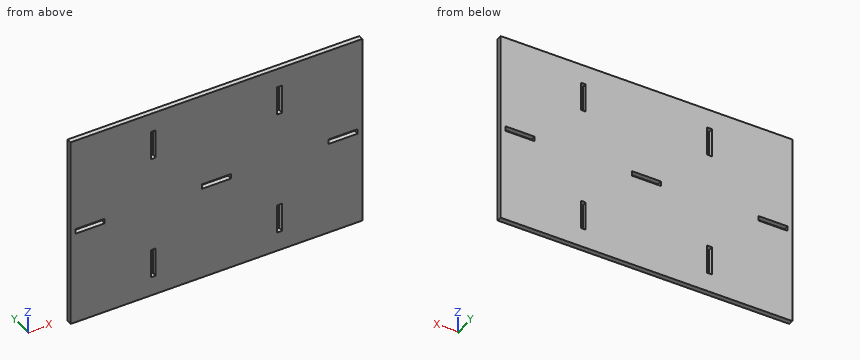
```python
from build123d import *

# Parameters (mm, degrees)
SKETCH1_W           = 300
SKETCH1_H           = 200
BOSS_EXTRUDE1_DEPTH = 5
SKETCH2_W           = 30
SKETCH2_H           = 5
SKETCH2_W_2         = 5
SKETCH2_H_2         = 30
CUT_EXTRUDE1_DEPTH  = 5


with BuildPart() as part:
    # Sketch1 → Boss-Extrude1 (new body)
    with BuildSketch(Plane(origin=(0, 0, 0), x_dir=(1, 0, 0), z_dir=(0, 1, 0))):
        Rectangle(SKETCH1_W, SKETCH1_H)
    extrude(amount=BOSS_EXTRUDE1_DEPTH)

    # Sketch2 → Cut-Extrude1 (cut)
    with BuildSketch(Plane(origin=(0, 5, 0), x_dir=(1, 0, 0), z_dir=(0, 1, 0))):
        with Locations((-130, 0)):
            Rectangle(SKETCH2_W, SKETCH2_H)
        with Locations((130, 0)):
            Rectangle(SKETCH2_W, SKETCH2_H)
        with Locations((-65, 65)):
            Rectangle(SKETCH2_W_2, SKETCH2_H_2)
        with Locations((-65, -65)):
            Rectangle(SKETCH2_W_2, SKETCH2_H_2)
        with Locations((65, 65)):
            Rectangle(SKETCH2_W_2, SKETCH2_H_2)
        with Locations((65, -65)):
            Rectangle(SKETCH2_W_2, SKETCH2_H_2)
        Rectangle(SKETCH2_W, SKETCH2_H)
    extrude(amount=-CUT_EXTRUDE1_DEPTH, mode=Mode.SUBTRACT)


solid = part.part
```
Geometry check sheet. Reference: the model listing, model coordinates, mm. Coordinates: 2 decimals unless noted, no trailing zeros. Order: outer loops, then holes, each group sorted by start corner. A loop starts at its lowest first (then second) coordinate and runs counter-clockwise, first axis right, second up. Notation, with made-up numbers: M -8.5,41 L 18.5,41 A18 ccw 18.5,74 Z; hole C 7.5,-21.5 d6. An arc over 180 degrees is marked long. One line per question, with ' | ' between items. Start each with the question number.
Item 1: Material ranges on L1, parallel to X at y = 2.9, z = 62; L2, parallel to X at y = 1.95, z = 1; L3, parallel to Z at x = -7.5, y = 3.9, recorded low to high. Write a range as [from, to].
Item 2: Cross-section at A-A on x = -130.5. Enter the section's corners in (y, z).
Item 3: Cross-section at B-B on y = 2.1. State how many separate pieces and enclosed holes the cut face has, then the cut area to 4 significant figures.
Findings:
1) L1: x = [-150, -67.5], [-62.5, 62.5], [67.5, 150] | L2: x = [-150, -145], [-115, -15], [15, 115], [145, 150] | L3: z = [-100, -2.5], [2.5, 100]
2) outline: M 0,-100 L 5,-100 L 5,-2.5 L 0,-2.5 Z; M 0,2.5 L 5,2.5 L 5,100 L 0,100 Z
3) separate pieces: 1 | enclosed holes: 7 | area: 58,950 mm²
